Input: part model. Units: mm. Frame: model coordinates. Give positions to 0.01 mm unless a question says otherwise; leave off trailing zeros. Order: outer loops, then holes, each group sorted by start corner. A loop starts at its lowest first (then second) coordinate and runs counter-clockwise, first axis right, second up. Notation, with made-up numbers: (77, -32) - (117, -32) arc R21 ccw to (117, 0) - close; hole circle Ø4 at (-35, 22). An arc over 180 degrees is marked (long way). Answer in a Markdown table with one row per item. Add a question column.
1. Contact query for flat-ended pins moving along their axis: pin 1 (4 mm diameter, centred on x = -7.5, y = -0.5, fed in from +Z) (3 decimals); pin 2 (5 mm diameter, centred on y = 10, z = 15.5, fed in from -X); pin 3 (1.5 mm diameter, centred on y = -9, z = 30, fed in from +X). Output: stop coordinate, or through.
2. Ray query, line 1 (Y direction, x = 0, z = 59.5); line 2 (Z direction, x = -3.75, y = -3.5) (3 decimals); line 3 (X direction, y = -8.25, z = 89). Return the intervals inside material, ascending. Write a range as [from, to].
3. Section query C-C on z = 79. Return loops of the section in (x, y) (1 decimal), and give its area (3 significant figures).
4. Mould query, pull axis X, two halves, no side actions, for faces 1 (the face through (0, 0, 0)), 2 (the face through (-14.274, 0.628, 48.246)), 3 (the face through (0, 0, 3.175)), 4 (the face through (10.6, 3.34, 49.86)). Classes: released by +X, released by -X, zero draft, split by the parting line, or undercut.
```python
from build123d import *

# Parameters (mm, degrees)
SKETCH1_R           = 14.2875
BOSS_EXTRUDE1_DEPTH = 95.25
SKETCH2_R           = 11.1125
CUT_EXTRUDE1_DEPTH  = 92.075
FILLET1_R           = 2.54


with BuildPart() as part:
    # Sketch1 → Boss-Extrude1 (new body)
    with BuildSketch(Plane.XY):
        Circle(SKETCH1_R)
    extrude(amount=BOSS_EXTRUDE1_DEPTH)

    # Sketch2 → Cut-Extrude1 (cut)
    with BuildSketch(Plane.XY.offset(95.25)):
        Circle(SKETCH2_R)
    extrude(amount=-CUT_EXTRUDE1_DEPTH, mode=Mode.SUBTRACT)

    # Fillet1
    fillet1_edges = [part.edges().sort_by_distance(p)[0] for p in [
        (-14.2875, 0, 0),
    ]]
    fillet(fillet1_edges, radius=FILLET1_R)


solid = part.part
```
Answer:
| question | item | result |
|---|---|---|
| 1 | pin 1 | stops at z = 3.175 |
| 1 | pin 2 | stops at x = -12.16 |
| 1 | pin 3 | stops at x = 11.66 |
| 2 | line 1 | y = [-14.29, -11.11], [11.11, 14.29] |
| 2 | line 2 | z = [0, 3.175] |
| 2 | line 3 | x = [-11.66, -7.44], [7.44, 11.66] |
| 3 | outline | circle Ø28.6 at (0, 0); hole circle Ø22.2 at (0, 0) |
| 3 | area | 253 mm² |
| 4 | face 1 | zero draft |
| 4 | face 2 | split by the parting line |
| 4 | face 3 | undercut |
| 4 | face 4 | undercut |
